```python
from build123d import *

# Parameters (mm, degrees)
SKETCH_1_R          = 25
SKETCH_1_R_2        = 2
SKETCH_1_R_3        = 4
EXTRUDE_1_DEPTH     = 3
SKETCH_2_R          = 12
EXTRUDE_2_DEPTH     = 10
CUT_EXTRUDE_START   = -24
CUT_EXTRUDE_1_DEPTH = 24
SKETCH_4_R          = 2
CUT_EXTRUDE_2_DEPTH = 19


with BuildPart() as part:
    # 草图1 → 凸台-拉伸1 (new body)
    with BuildSketch(Plane.XY):
        Circle(SKETCH_1_R)
        with Locations((0, 19)):
            Circle(SKETCH_1_R_2, mode=Mode.SUBTRACT)
        with Locations((13.435028843, 13.435028843)):
            Circle(SKETCH_1_R_2, mode=Mode.SUBTRACT)
        with Locations((19, 0)):
            Circle(SKETCH_1_R_2, mode=Mode.SUBTRACT)
        with Locations((13.435028843, -13.435028843)):
            Circle(SKETCH_1_R_2, mode=Mode.SUBTRACT)
        with Locations((0, -19)):
            Circle(SKETCH_1_R_2, mode=Mode.SUBTRACT)
        with Locations((-13.435028843, -13.435028843)):
            Circle(SKETCH_1_R_2, mode=Mode.SUBTRACT)
        with Locations((-19, 0)):
            Circle(SKETCH_1_R_2, mode=Mode.SUBTRACT)
        with Locations((-13.435028843, 13.435028843)):
            Circle(SKETCH_1_R_2, mode=Mode.SUBTRACT)
        Circle(SKETCH_1_R_3, mode=Mode.SUBTRACT)
    extrude(amount=EXTRUDE_1_DEPTH)

    # 草图2 → 凸台-拉伸2 (add)
    with BuildSketch(Plane.XY.offset(3)):
        Circle(SKETCH_2_R)
    extrude(amount=EXTRUDE_2_DEPTH)

    # 草图3 → 切除-拉伸1 (cut)
    with BuildSketch(Plane.XY.offset(13).offset(CUT_EXTRUDE_START)):
        with BuildLine():
            Line((-3.464101615, -2), (3.464101615, -2))
            ThreePointArc((3.464101615, -2), (0, 4), (-3.464101615, -2))
        make_face()
    extrude(amount=CUT_EXTRUDE_1_DEPTH, mode=Mode.SUBTRACT)

    # 草图4 → 切除-拉伸2 (cut)
    with BuildSketch(Plane(origin=(0, -2, 0), x_dir=(1, 0, 0), z_dir=(0, 1, 0))):
        with Locations(Location((0, -8, 0), (0, 0, 90))):
            Circle(SKETCH_4_R)
    extrude(amount=CUT_EXTRUDE_2_DEPTH, mode=Mode.SUBTRACT)


solid = part.part
```
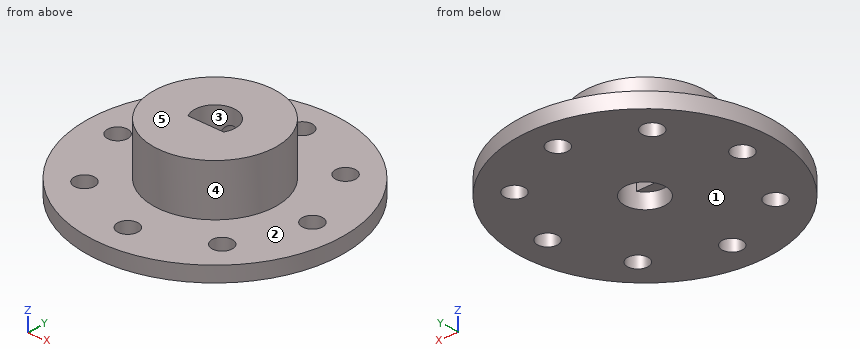
Build history of the part. All positions in model axes, mm. Face numbers are marked on the shaded views. A direction names the side the tool comes from. Coordinates: 2 decimals unless noted, no trailing zeros. Order: outer loops, then holes, each group sorted by start corner. A loop starts at its lowest first (then second) coordinate and runs counter-clockwise, first axis right, second up.
Item 1: Saw through at A-A on x = 0. List the corners of the cut face in (y, z), then the cut area to 3 significant figures.
Filled in:
outline: (-25, 0) - (-21, 0) - (-21, 3) - (-25, 3) - close; (-17, 0) - (-4, 0) - (-4, 3) - (-2, 3) - (-2, 13) - (-12, 13) - (-12, 3) - (-17, 3) - close; (4, 0) - (17, 0) - (17, 3) - (12, 3) - (12, 6) - (4, 6) - close; (4, 10) - (12, 10) - (12, 13) - (4, 13) - close; (21, 0) - (25, 0) - (25, 3) - (21, 3) - close
area: 250 mm2
Item 2: Drill centre lines: L1, parallel to Y at x = 0, z = 0.9; L2, parallel to Y at x = 0, z = 10.25; L3, parallel to Z at x = 16.5, y = 4.5. Where is each one in solid material? Low to high.
Filled in:
L1: y = -25 to -21, -17 to -4, 4 to 17, 21 to 25
L2: y = -12 to -2, 4 to 12
L3: z = 0 to 3
Item 3: Saw through at D-D on y = 19. List the corners of the cut face in (x, z).
Filled in:
outline: (-16.25, 0) - (-2, 0) - (-2, 3) - (-16.25, 3) - close; (2, 0) - (16.25, 0) - (16.25, 3) - (2, 3) - close
Item 4: Saw through at B-B on y = 0. List the corners of the cut face in (x, z), then the cut area to 3 significant figures.
Filled in:
outline: (-25, 0) - (-21, 0) - (-21, 3) - (-25, 3) - close; (-17, 0) - (-4, 0) - (-4, 13) - (-12, 13) - (-12, 3) - (-17, 3) - close; (4, 0) - (17, 0) - (17, 3) - (12, 3) - (12, 13) - (4, 13) - close; (21, 0) - (25, 0) - (25, 3) - (21, 3) - close
area: 262 mm2
Item 5: Drop flat-ended pins along their axis: pin 1 Ø5 at (x, y) = (-19, 0) entering from +Z; pin 2 Ø5.5 at (x, z) = (1.5, 8.5) entering from +Y; pin 3 Ø2.5 at (x, y) = (13.44, -13.44) entering from -Z; pin 4 Ø1.5 at (y, z) = (2, 10.5) entering from +X. Give the stop position or say it passes through.
Filled in:
pin 1: stops at z = 3
pin 2: stops at y = 12
pin 3: passes through
pin 4: stops at x = 11.93
Item 6: Saw through at C-C on z = 1.25. State how many separate pieces and enclosed holes the cut face has, then the cut area to 3 significant figures.
Filled in:
separate pieces: 1
enclosed holes: 9
area: 1,810 mm2
Item 7: Tool access for the marked faces 1 and 2: list every direction of +Z, -Z, +X, -X, +Y, -Y with a clear straight run to the whole face (end or side of a thin tool).
Filled in:
face 1: -Z, +X, -X, +Y, -Y
face 2: +Z
Item 8: Mould opens along X. For the marked faces 3, 4 and 5 say: released by +X, released by -X, zero draft, split by the parting line, or undercut.
Filled in:
face 3: undercut
face 4: split by the parting line
face 5: zero draft
